Source: CAD feature listing. Evaluate the final solid. Frame: model axes, mm. A direction names the side the tool comes from. Round coordinates to 2 decimals unless told otherwise and drop trailing zeros. Write each loop counter-clockwise with the first axis right and the second up, starting at its lowest first coordinate (ties: lowest second). Pieces come first, ordered by that corner, then holes. Notation, with made-up numbers: M -37,65 L -25,65 A19 ccw -25,88 Z; hole C 50.25,2.25 d2. An arc over 180 degrees is marked long. Put each result on its own line as item: value. Start each with the question number.
Autodesk Inventor part; units mm, degrees
ref_plane "YZ Plane" through (0, 0, 0) normal (1, 0, 0) x (0, 1, 0)
ref_plane "XZ Plane" through (0, 0, 0) normal (0, 1, 0) x (-1, 0, 0)
ref_plane "XY Plane" through (0, 0, 0) normal (0, 0, 1) x (1, 0, 0)
sketch "Sketch1" plane through (0, 0, 0) normal (1, 0, 0) x (0, 1, 0)
  line L0 (0, 20) -> (15, 20)
  line L1 (15, 20) -> (15, 12)
  line L2 (15, 12) -> (35, 12)
  line L3 (35, 12) -> (35, 0)
  line L4 (35, 0) -> (0, 0)
  line L5 (0, 0) -> (0, 20)
  dimension "d0" = 35
  dimension "d30" = 20
  dimension "d31" = 8
  dimension "d33" = 20
extrude "Extrusion1" add sketch "Sketch1" along normal mid plane 50
sketch "Sketch2" plane through (-25, 0, 0) normal (0, -1, 0) x (1, 0, 0)
  line L0 (0, 20) -> (12.5, 20)
  line L1 (12.5, 20) -> (12.5, 12)
  line L2 (12.5, 12) -> (0, 12)
  line L3 (0, 12) -> (0, 20)
  line L4 (37.5, 20) -> (50, 20)
  line L5 (50, 20) -> (50, 12)
  line L6 (50, 12) -> (37.5, 12)
  line L7 (37.5, 12) -> (37.5, 20)
  line L8 (0, 20) -> (50, 20)
  line L9 (50, 12) -> (0, 12)
  dimension "d15" = 25
extrude "Extrusion2" cut sketch "Sketch2" against normal through all contours L0 L1 L2 L3 | L4 L5 L6 L7
sketch "Sketch4" plane through (-25, 35, 12) normal (0, 0, 1) x (1, 0, 0)
  line L0 (6, -29) -> (6, -12) construction
  line L1 (9.25, -29) -> (9.25, -12)
  line L2 (2.75, -12) -> (2.75, -29)
  arc A0 (2.75, -29) -> (9.25, -29) centre (6, -29) ccw
  arc A1 (9.25, -12) -> (2.75, -12) centre (6, -12) ccw
  line L3 (12.5, -35) -> (0, -35)
  line L4 (0, -35) -> (0, 0)
  point P0 (6, -20.5)
  dimension "d24" = 6.5
  dimension "d25" = 17
  dimension "d38" = 6
  dimension "d39" = 6
extrude "Extrusion3" cut sketch "Sketch4" against normal through all
mirror "Mirror1" about plane through (0, 0, 0) normal (1, 0, 0) of "Extrusion3"
sketch "Sketch5" plane through (-25, 0, 0) normal (0, -1, 0) x (1, 0, 0)
  line L0 (12.5, 20) -> (37.5, 20)
  point P0 (25, 0)
  point P1 (25, 16)
  point P2 (25, 20)
  dimension "d40" = 4
hole "Hole1" at (0, 0, 16) direction (0, 1, 0) diameter 4.134 end through all
properties part number "Clamping Block" material "Aluminum 6061"
(1) Section query B-B (x = 0). Return loops of the section in (y, z).
(2) Access query for faces 1 (the flat face through (-12.5, 7, 16)), 2 (the flat face through (22.25, 14, 6)), 3 (the flat face through (12.5, 7, 16)). Directions: +Z, -Z, +X, -X, +Y, -Y. A direction counts if a zero-diameter tool reaches every point of the face in a straight line with its end or side. Return the directions, or none.
(3) Ray query, line 1 along X through (y, z) = (7.5, 7.75); line 2 along X through (y, z) = (8, 16); line 3 along X through (y, z) = (3, 6.5). Return the intervals inside material, ascending.
(4) Contact query for flat-ended pins moving along their axis: P1, Ø5, axis at x = -16, y = 12, coming from the +Z side; P2, Ø4, axis at y = 9.5, z = 17, coming from the +X side. Output: stop coordinate, or through.
(5) Section query A-A (y = 18). Return loops of the section in (x, z).
(6) Pull-direction query (Y, two-part tool) for faces 4 (the flat face through (0, 0, 8)), 5 (the cylindrical face through (18.93, 2.75, 6.08)), 6 (the flat face through (0, 7, 20)), 7 (the flat face through (0, 35, 6)); classes: +Y half, -Y half, draft (parallel to the pull), parting line (faces both ways), or undercut.
(7) Section query C-C (y = 5). Return loops of the section in (x, z), and give its area (3 significant figures).
(8) Section query D-D (z = 1.5). Return loops of the section in (x, y).
Entries:
1. outline: M 0,0 L 35,0 L 35,12 L 15,12 L 15,13.93 L 0,13.93 Z; M 0,18.07 L 15,18.07 L 15,20 L 0,20 Z
2. face 1: +Z, -X, +Y, -Y
2. face 2: +Z, -Z
2. face 3: +Z, +X, +Y, -Y
3. line 1: -25 to -22.25, -15.75 to 15.75, 22.25 to 25
3. line 2: -12.5 to -2.07, 2.07 to 12.5
3. line 3: -25 to -20.25, -17.75 to 17.75, 20.25 to 25
4. P1: z = 12
4. P2: x = 12.5
5. outline: M -25,0 L -22.25,0 L -22.25,12 L -25,12 Z; M -15.75,0 L 15.75,0 L 15.75,12 L -15.75,12 Z; M 22.25,0 L 25,0 L 25,12 L 22.25,12 Z
6. face 4: -Y half
6. face 5: undercut
6. face 6: draft
6. face 7: +Y half
7. outline: M -25,0 L -22.09,0 L -22.09,12 L -25,12 Z; M -15.91,0 L 15.91,0 L 15.91,12 L 12.5,12 L 12.5,20 L -12.5,20 L -12.5,12 L -15.91,12 Z; M 22.09,0 L 25,0 L 25,12 L 22.09,12 Z; hole C 0,16 d4.13
7. area: 638 mm2
8. outline: M -25,0 L 25,0 L 25,35 L -25,35 Z; hole M -22.25,6 A3.25 ccw -15.75,6 L -15.75,23 A3.25 ccw -22.25,23 Z; hole M 15.75,6 A3.25 ccw 22.25,6 L 22.25,23 A3.25 ccw 15.75,23 Z
